Read the model definition and answer for the solid it produces. Units are mm, in the model's axes. A direction names the side the tool comes from. Coordinates: 2 decimals unless noted, no trailing zeros. Write each loop counter-clockwise with the first axis right and the second up, starting at its lowest first coordinate (ties: lowest second). Pieces come first, ordered by that corner, then holes. Notation, with made-up numbers: (1.5, 56) -> (10.5, 56) arc R17 ccw to (10.5, 74) -> close; hole circle Ø1 at (78.5, 66.5). An arc over 180 degrees is marked (long way). Use CSV: the item, a comma, the result in double quotes.
from build123d import *

# Parameters (mm, degrees)
F0_W     = 40.8606864512
F0_H     = 43.7535122037
F1_DEPTH = 600
F2_DEPTH = 600
F3_DEPTH = 2200
F4_T     = -18


with BuildPart() as f1:
    # F0 (on Right) → F1 (new body)
    with BuildSketch(Plane.YZ):
        with Locations((-20.4303432256, 21.8767561018)):
            Rectangle(F0_W, F0_H)
    extrude(amount=F1_DEPTH)

    # F2 (add): a face of the model
    f2_faces = [f1.faces().sort_by_distance(p)[0] for p in [
        (300, 0, 21.8767561018),
    ]]
    extrude(f2_faces, amount=-F2_DEPTH)

    # F3 (add): a face of the model
    f3_faces = [f1.faces().sort_by_distance(p)[0] for p in [
        (300, -300, 0),
    ]]
    extrude(f3_faces, amount=-F3_DEPTH)

    # F4
    f4_openings = [f1.faces().sort_by_distance(p)[0] for p in [
        (0, -300, 1100),
    ]]
    offset(amount=F4_T, openings=f4_openings)


solid = f1.part
1. Find the intervals of material crossed by line 1 along Y through (x, z) = (213, 1896); line 2 along Z through (x, y) = (425, -100.5); line 3 along X through (y, z) = (-386, 394), in increasing order.
Solutions:
line 1,"y = -600 to -582, -18 to 0"
line 2,"z = 0 to 18, 2182 to 2200"
line 3,"x = 582 to 600"
2. Each of these flat-tipped pins is pushed along its axis until it touches: pin 1 Ø1.5 at (y, z) = (-164.5, 1189) entering from -X; pin 2 Ø1 at (x, z) = (114.5, 1346) entering from +Y. Where does it stop, or does it pass through?
Solutions:
pin 1,"stops at x = 582"
pin 2,"stops at y = 0"
3. For a pull along Y with two mould halves and no side action, classify faces 1 (the flat face through (296, 0, 1085)), 2 (the flat face through (287, -296, 2182)), 3 (the flat face through (296, -600, 1085)), 4 (the flat face through (296, -296, 0)) as pulls with the +Y half, pulls with the -Y half, needs draft (parallel to the pull), parting line crosses it, or undercut.
Solutions:
face 1,"pulls with the +Y half"
face 2,"undercut"
face 3,"pulls with the -Y half"
face 4,"needs draft"
4. A cutting plane is placed at A-A (x = 268.5). Give the vertices of the cut face in (y, z), and give its area (3 significant figures).
Solutions:
outline,"(-600, 0) -> (0, 0) -> (0, 2200) -> (-600, 2200) -> close; hole (-582, 18) -> (-18, 18) -> (-18, 2182) -> (-582, 2182) -> close"
area,"99,500 mm^2"
5. A cutting plane is placed at C-C (z = 1005). Give the vertices of the cut face in (x, y).
Solutions:
outline,"(0, -600) -> (600, -600) -> (600, 0) -> (0, 0) -> (0, -18) -> (582, -18) -> (582, -582) -> (0, -582) -> close"
6. A tool of negligible diameter and unlimited length cuts with its end or side. For faces 5 (the flat face through (296, -296, 2200)), 6 (the flat face through (287, -296, 18)), from which of +Z, -Z, +X, -X, +Y, -Y can it reach the whole face along a straight path? Write none if from no direction.
Solutions:
face 5,"+Z, +X, -X, +Y, -Y"
face 6,"-X"
7. A cutting plane is placed at B-B (y = -338.5). Give the vertices of the cut face in (x, z).
Solutions:
outline,"(0, 0) -> (600, 0) -> (600, 2200) -> (0, 2200) -> (0, 2182) -> (582, 2182) -> (582, 18) -> (0, 18) -> close"
